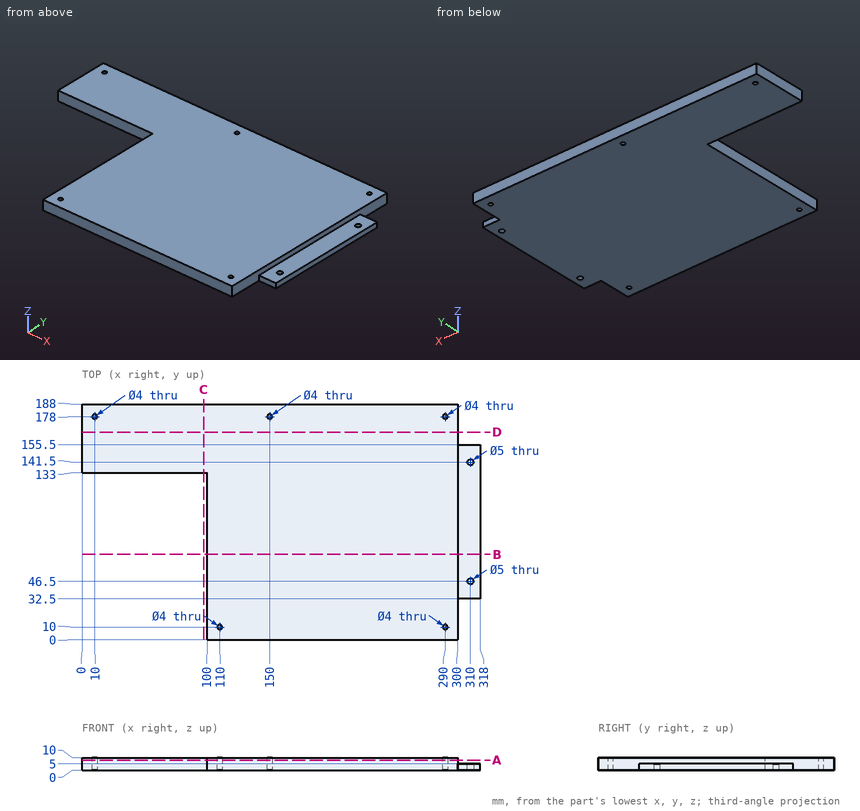
Geometry check sheet. Reference: drawing and pictorial views, mm from the part's lowest x, y, z. Coordinates: 2 decimals unless noted, no trailing zeros. Write each loop counter-clockwise with the first axis right and the second up, starting at its lowest first coordinate (ties: lowest second). Pieces come first, ordered by that corner, then holes. Notation, with made-up numbers: M 77.5,69.25 L 124.5,69.25 A18 ccw 124.5,91.25 Z; hole C -35.5,-21.5 d1. An arc over 180 degrees is marked long. Write item = value, one per line. Start each with the question number.
1. Sectioned sample at B-B (y = 68). Record the cut outline in (x, z).
2. Go/stop test with flat-tipped pins: pin 1 (3 mm diameter, centred on y = 61, z = 6.5, fed in from -X); pin 2 (6 mm diameter, centred on x = 310, y = 46.5, fed in from -Z); pin 3 (4 mm diameter, centred on y = 117, z = 8, fed in from +X); pin 4 (9 mm diameter, centred on x = 311.5, y = 96, fed in from +Z). Record where each tip stops, or that it passes through.
3. Sectioned sample at A-A (z = 8). Record the cut outline in (x, y), then the cut area to 3 significant figures.
4. Thickness scan on probe 1 along Y at (x, z) = (310, 2.9); probe 2 along X at (y, z) = (178, 6.5); probe 3 along X at (y, z) = (10.5, 3.5). Record the ranges inside material, lowest first.
5. Sectioned sample at D-D (y = 165.5). Record the cut outline in (x, z).
6. Sectioned sample at C-C (x = 97). Record the cut outline in (y, z), then the cut area to 3 significant figures.
The answers:
q1.outline = M 100,0 L 318,0 L 318,5 L 300,5 L 300,10 L 100,10 Z
q2.pin_1 = 100
q2.pin_2 = 0
q2.pin_3 = 300
q2.pin_4 = 5
q3.outline = M 0,133 L 100,133 L 100,0 L 300,0 L 300,188 L 0,188 Z; hole C 10,178 d4; hole C 110,10 d4; hole C 150,178 d4; hole C 290,10 d4; hole C 290,178 d4
q3.area = 43,000 mm²
q4.probe_1 = 32.5 to 44, 49 to 139, 144 to 155.5
q4.probe_2 = 0 to 8, 12 to 148, 152 to 288, 292 to 300
q4.probe_3 = 100 to 108.06, 111.94 to 288.06, 291.94 to 300
q5.outline = M 0,0 L 300,0 L 300,10 L 0,10 Z
q6.outline = M 133,0 L 188,0 L 188,10 L 133,10 Z
q6.area = 550 mm²
